CAD build for the part. Positions are in the model's coordinates, mm. Face numbers are marked on the shaded views. Coordinates: 2 decimals unless noted, no trailing zeros. Order: outer loops, then holes, each group sorted by start corner. A loop starts at its lowest first (then second) coordinate and runs counter-clockwise, first axis right, second up.
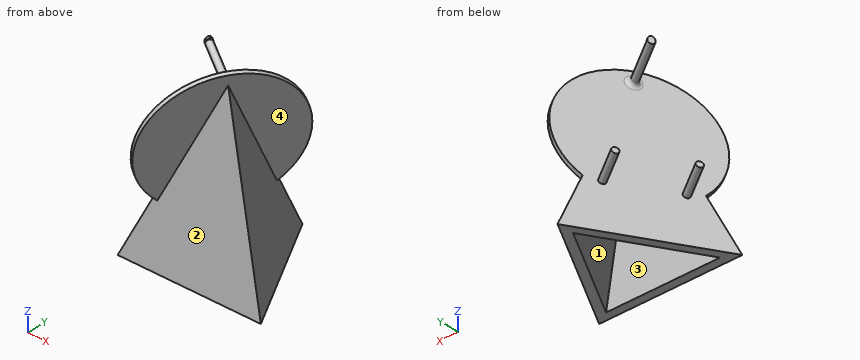
from build123d import *

# Parameters (mm, degrees)
AUFSATZ_LINEAR_AUSTRAGEN1_DEPTH = 40
FASE1_SIZE                      = 40
FASE1_SIZE_2                    = 9.973120114
WANDUNG1_T                      = -2
SKIZZE2_R                       = 17
AUFSATZ_LINEAR_AUSTRAGEN2_DEPTH = 1
SKIZZE3_R                       = 0.8
AUFSATZ_LINEAR_AUSTRAGEN3_DEPTH = 11
VERRUNDUNG1_R                   = 1
SKIZZE4_R                       = 0.8
AUFSATZ_LINEAR_AUSTRAGEN4_DEPTH = 8
AUFSATZ_LINEAR_START            = -0.5
AUFSATZ_LINEAR_AUSTRAGEN5_DEPTH = 0.5


with BuildPart() as part:
    # Skizze1 → Aufsatz-Linear austragen1 (new body)
    with BuildSketch(Plane.XY):
        Polygon((0, 30.310889132), (-17.5, 0), (17.5, 0), align=None)
    extrude(amount=AUFSATZ_LINEAR_AUSTRAGEN1_DEPTH)

    # Fase1
    # the kernel refuses this chamfer: 40, 9.973120114 mm, written as the material it takes off along each edge
    with BuildSketch(Plane(origin=(-121.385689972, 0, 40), x_dir=(0, -0.009314926653100153, -0.9999566151296001), z_dir=(1, 0, 0)), Plane(origin=(69.442844986, -89.967646606, 40), x_dir=(0.008066963115973384, 0.004657463326550014, -0.9999566151296001), z_dir=(-0.5, 0.8660254037844387, 0)), Plane(origin=(51.942844986, 120.278535738, 40), x_dir=(-0.008066963115973531, 0.0046574633265501, -0.9999566151296001), z_dir=(-0.5, -0.8660254037844387, 0))) as fase1_piece_1:
        Polygon((FASE1_SIZE * 0.99995661513, FASE1_SIZE * 0.0093149266531), (-FASE1_SIZE_2 * 0.00931492665285, FASE1_SIZE_2 * 0.999956615102), (0, 0), align=None)
    extrude(amount=242.771379945, mode=Mode.SUBTRACT)

    # Wandung1
    wandung1_openings = [part.faces().sort_by_distance(p)[0] for p in [
        (0, 10.103629711, 0),
    ]]
    offset(amount=WANDUNG1_T, openings=wandung1_openings, kind=Kind.INTERSECTION)

    # Skizze2 → Aufsatz-Linear austragen2 (add)
    with BuildSketch(Plane(origin=(-12.356843578, 7.134226966, 3.557525123), x_dir=(0.20951050732099702, -0.1209609477998327, 0.9702957262759971), z_dir=(-0.8403007481384855, 0.4851478631379986, 0.2419218955996654))):
        with Locations((22.558111296, 8.75)):
            Circle(SKIZZE2_R)
    extrude(amount=-AUFSATZ_LINEAR_AUSTRAGEN2_DEPTH)

    # Skizze3 → Aufsatz-Linear austragen3 (add)
    with BuildSketch(Plane(origin=(-12.356843578, 7.134226966, 3.557525123), x_dir=(0.20951050732099702, -0.1209609477998327, 0.9702957262759971), z_dir=(-0.8403007481384855, 0.4851478631379986, 0.2419218955996654))):
        with Locations(Location((36.558111296, 8.75, 0), (0, 0, 270))):
            Circle(SKIZZE3_R)
    extrude(amount=AUFSATZ_LINEAR_AUSTRAGEN3_DEPTH)

    # Verrundung1
    verrundung1_edges = [part.edges().sort_by_distance(p)[0] for p in [
        (0.077464866, 10.98266578, 39.029704274),
    ]]
    fillet(verrundung1_edges, radius=VERRUNDUNG1_R)

    # Skizze4 → Aufsatz-Linear austragen4 (add)
    with BuildSketch(Plane(origin=(-12.356843578, 7.134226966, 3.557525123), x_dir=(0.20951050732099705, -0.12096094779983271, 0.9702957262759971), z_dir=(-0.8403007481384855, 0.4851478631379987, 0.24192189559966543))):
        with Locations(Location((9.558111296, 16.75, 0), (0, 0, 270))):
            Circle(SKIZZE4_R)
        with Locations(Location((9.558111296, 0.75, 0), (0, 0, 270))):
            Circle(SKIZZE4_R)
    extrude(amount=AUFSATZ_LINEAR_AUSTRAGEN4_DEPTH)

    # Skizze5 → Aufsatz-Linear austragen5 (add)
    with BuildSketch(Plane(origin=(-21.600151808, 12.470853461, 6.218665974), x_dir=(0.209510507320997, -0.1209609477998327, 0.9702957262759971), z_dir=(-0.8403007481384855, 0.4851478631379987, 0.24192189559966537)).offset(AUFSATZ_LINEAR_START)):
        with BuildLine():
            ThreePointArc((36.558111296, 9.55), (35.758111296, 8.75), (36.558111296, 7.95))
            add(Edge.make_bspline(
                [(36.558111296, 7.95), (37.758111296, 7.95), (37.758111296, 8.75), (37.758111296, 9.55), (36.558111296, 9.55)],
                knots=[4.71238898, 4.71238898, 4.71238898, 6.283185307, 6.283185307, 7.853981634, 7.853981634, 7.853981634], degree=2, weights=[1, 0.707106781, 1, 0.707106781, 1]))
        make_face()
    extrude(amount=AUFSATZ_LINEAR_AUSTRAGEN5_DEPTH)


solid = part.part
1) Slice it at B-B (x = 10). List the corners of the cut face in (y, z), plus the area to 3 significant figures.
2) Slice it at A-A (z = 10). List the corners of the cut face in (x, y).
3) Slice it at C-C (y = 28.5). List the corners of the cut face in (x, z), plus the area to 3 significant figures.
4) Pin check, flat tips, straight feed: P1, Ø8, axis at y = 26, z = 26, coming from the -X side; P2, Ø8, axis at x = -5.5, z = 37, coming from the +Y side; P3, Ø8, axis at y = 24.5, z = 27.5, coming from the +X side. Stop position of each tip, or through.
5) Two-plate mould, pull along X, no slides. Class the marked faces 1, 2, 3 and 4: released by +X, released by -X, zero draft, split by the parting line, or undercut.
6) Drill centre lines: probe 1 along X at (y, z) = (16, 12.5); probe 2 along Y at (x, z) = (-4.5, 7); probe 3 along X at (y, z) = (7.5, 17). Where is each one in solid material? Low to high.
7) Slice it at D-D (z = 4). List the corners of the cut face in (x, y).
Worked out:
1. outline: (0, 0) - (2.06, 0) - (4.33, 9.1) - (8.87, 0) - (12.99, 0) - (4.33, 17.37) - close
1. area: 81.8 mm2
2. outline: (-13.18, 2.49) - (13.18, 2.49) - (0, 25.32) - close; hole (-9.61, 4.55) - (9.61, 4.55) - (0, 21.2) - close
3. outline: (-1.05, 0) - (1.05, 0) - (0, 3.63) - close
3. area: 3.80 mm2
4. P1: stops at x = 2.42
4. P2: stops at y = 15.01
4. P3: stops at x = 6.8
5. face 1: undercut
5. face 2: zero draft
5. face 3: undercut
5. face 4: released by +X
6. probe 1: x = -4.66 to -2.28, 2.28 to 4.66
6. probe 2: y = 1.75 to 3.81, 14.9 to 19.03
6. probe 3: x = -8.28 to -5.9, 5.9 to 8.28
7. outline: (-15.77, 1) - (15.77, 1) - (0, 28.32) - close; hole (-12.2, 3.06) - (12.2, 3.06) - (0, 24.19) - close
